Could you check a few things on this drawing? It's one solid part, dimensions in mm from its lowest x, y, z. Give positions to 0.01 mm unless a question says otherwise; leave off trailing zeros. Order: outer loops, then holes, each group sorted by start corner. A loop starts at its lowest first (then second) coordinate and runs counter-clockwise, first axis right, second up. Notation, with made-up numbers: M 27,65.25 L 35,65.25 A17 ccw 35,74.25 Z; hole C 77.25,-22 d4. An arc over 180 degrees is marked long. Use one line per item in the form item = value. Start each with the question number.
1. I want a section at A-A, the plane z = 610. List the corners of the cut face in (x, y) for me.
2. We'd pull the mould along Z, two halves only. Please class the marked faces 1 and 2: +Z half, -Z half, draft (parallel to the pull), parting line (faces both ways), or undercut.
3. I want a section at C-C, the plane x = 46.5. List the corners of the cut face in (y, z) for me (1 decimal).
4. Will these pins go through, and if not, where does the flat tip stop? P1, Ø5, axis at x = 69.5, y = 229.5, coming from the +Z side; P2, Ø22.5, axis at x = 38, y = 722.5, coming from the +Z side; P3, Ø10, axis at x = 57.5, y = 746.5, coming from the -Z side.
5. I need wall thicknesses on L1, parallel to Y at x = 57, z = 960; L2, parallel to Y at x = 36, z = 622; L3, parallel to X at y = 1083, z = 234. Which ranges of each line are inside material? Lowest first, please.
6. I want a section at B-B, the plane y = 610. List the corners of the cut face in (x, z) for me.
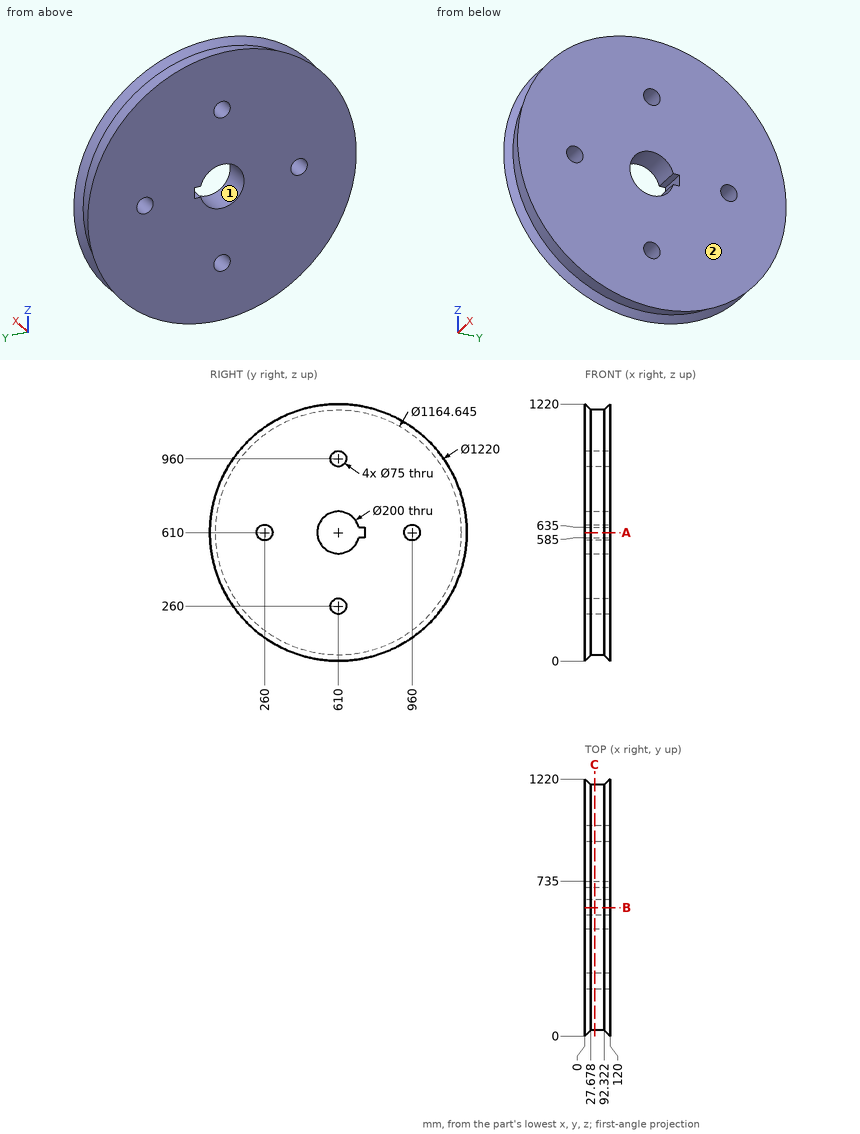
Check result:
q1.outline = M 0,0 L 27.68,27.68 L 92.32,27.68 L 120,0 L 120,222.5 L 0,222.5 Z; M 0,297.5 L 120,297.5 L 120,510 L 0,510 Z; M 0,735 L 120,735 L 120,922.5 L 0,922.5 Z; M 0,997.5 L 120,997.5 L 120,1220 L 92.32,1192.32 L 27.68,1192.32 L 0,1220 Z
q2.face_1 = undercut
q2.face_2 = draft
q3.outline = C 610,610 d1164.6; hole C 260,610 d75; hole C 610,260 d75; hole C 610,960 d75; hole M 706.8,585 L 735,585 L 735,635 L 706.8,635 A100 ccw long Z; hole C 960,610 d75
q4.P1 = 1052.96
q4.P2 = 1183.45
q4.P3 = 42.72
q5.L1 = 144.6 to 572.5, 647.5 to 1075.4
q5.L2 = 27.8 to 224.47, 295.53 to 510.72, 735 to 924.47, 995.53 to 1192.2
q5.L3 = 0 to 5.76, 114.24 to 120
q6.outline = M 0,0 L 27.68,27.68 L 92.32,27.68 L 120,0 L 120,222.5 L 0,222.5 Z; M 0,297.5 L 120,297.5 L 120,510 L 0,510 Z; M 0,710 L 120,710 L 120,922.5 L 0,922.5 Z; M 0,997.5 L 120,997.5 L 120,1220 L 92.32,1192.32 L 27.68,1192.32 L 0,1220 Z
